Part model, mm, in its own coordinate system. A direction names the side the tool comes from. Give positions to 0.01 mm unless a question says otherwise; leave off trailing zeros. Order: outer loops, then holes, each group sorted by start corner. A loop starts at its lowest first (then second) coordinate and runs counter-clockwise, first axis right, second up. Notation, with made-up numbers: M 33.25,29.5 L 83.25,29.5 A17 ccw 83.25,35.5 Z; hole C -4,34 d6. An arc over 180 degrees is marked long. Answer as a JSON object with one key per item and string values.
from build123d import *

# Parameters (mm, degrees)
BOSS_EXTRUDE1_DEPTH = 2.54
SKETCH2_R           = 6.35
CUT_EXTRUDE1_DEPTH  = 2.54
SKETCH3_W           = 175.067056309
SKETCH3_H           = 2.54
BOSS_EXTRUDE2_DEPTH = 7.62
SKETCH4_W           = 175.067056309
SKETCH4_H           = 29.21
SKETCH4_W_2         = 164.016975536
SKETCH4_H_2         = 66.475239383
SKETCH4_W_3         = 84.822418372
SKETCH4_H_3         = 89.286756182
CUT_EXTRUDE2_DEPTH  = 2.54
FILLET1_R           = 12.7


with BuildPart() as part:
    # Sketch1 → Boss-Extrude1 (new body)
    with BuildSketch(Plane.XY.offset(-12.457776114)):
        Polygon((-175.067056309, 77.80274772), (129.732943691, 77.80274772), (129.732943691, 21.857628122), (0, 21.857628122), (0, -19.695936064), (-175.067056309, -19.695936064), align=None)
        with BuildLine():
            Line((-152.479240823, 20.309063936), (-5.464407031, 20.309063936))
            ThreePointArc((-5.464407031, 20.309063936), (-3.559407031, 18.404063936), (-5.464407031, 16.499063936))
            Line((-5.464407031, 16.499063936), (-152.479240823, 16.499063936))
            ThreePointArc((-152.479240823, 16.499063936), (-154.384240823, 18.404063936), (-152.479240823, 20.309063936))
        make_face(mode=Mode.SUBTRACT)
    extrude(amount=-BOSS_EXTRUDE1_DEPTH)

    # Sketch2 → Cut-Extrude1 (cut)
    with BuildSketch(Plane.XY.offset(-12.457776114)):
        with Locations((22.439796045, 50.825535486)):
            Circle(SKETCH2_R)
    extrude(amount=-CUT_EXTRUDE1_DEPTH, mode=Mode.SUBTRACT)

    # Sketch3 → Boss-Extrude2 (add)
    with BuildSketch(Plane.XY.offset(-12.457776114)):
        with Locations((-87.533528155, 26.024063936)):
            Rectangle(SKETCH3_W, SKETCH3_H)
        with Locations((-87.533528155, 10.784063936)):
            Rectangle(SKETCH3_W, SKETCH3_H)
    extrude(amount=BOSS_EXTRUDE2_DEPTH)

    # Sketch4 → Cut-Extrude2 (cut)
    with BuildSketch(Plane.XY.offset(-12.457776114)):
        with Locations((-87.533528155, -5.090936064)):
            Rectangle(SKETCH4_W, SKETCH4_H)
        with Locations((-93.058568541, 60.531683628)):
            Rectangle(SKETCH4_W_2, SKETCH4_H_2)
        with Locations((90.924098408, 47.502895008)):
            Rectangle(SKETCH4_W_3, SKETCH4_H_3)
    extrude(amount=-CUT_EXTRUDE2_DEPTH, mode=Mode.SUBTRACT)

    # Fillet1
    # the kernel refuses this fillet: 12.7 mm, written as the material it adds along each edge
    with BuildSketch(Plane(origin=(-11.050080773, 27.294063936, -12.457776114), x_dir=(0, 1, 0), z_dir=(0, 0, -1))) as fillet1_piece_1:
        with BuildLine():
            CenterArc((FILLET1_R, -FILLET1_R), FILLET1_R, 90, 90)
            Line((0, -FILLET1_R), (0, 0))
            Line((0, 0), (FILLET1_R, 0))
        make_face()
    extrude(amount=2.54)
    with BuildSketch(Plane(origin=(0, 21.857628122, 19.279716847), x_dir=(0, -1, 0), z_dir=(0, 0, -1))) as fillet1_piece_2_section:
        with BuildLine():
            CenterArc((12.7, -12.694997184), FILLET1_R, 91.608263763, 88.391736237)
            Line((0, -12.694997184), (0, 0))
            Line((0, 0), (12.343564187, 0))
        make_face()
    fillet1_piece_2 = extrude(amount=34.277492961, mode=Mode.PRIVATE)
    fillet1_piece_2 = split(fillet1_piece_2, bisect_by=Plane(origin=(0, 12.054063936, 19.279716847), z_dir=(0, -1, 0)), keep=Keep.TOP, mode=Mode.PRIVATE)
    fillet1_piece_2 = split(fillet1_piece_2, bisect_by=Plane(origin=(0, 21.857628122, -4.837776114), z_dir=(0, 0, -1)), keep=Keep.TOP, mode=Mode.PRIVATE)
    add(fillet1_piece_2)
    with BuildSketch(Plane(origin=(0, 21.857628122, -12.457776114), x_dir=(0, -1, 0), z_dir=(0, 0, -1))) as fillet1_piece_3:
        with BuildLine():
            CenterArc((12.7, -12.694997184), FILLET1_R, 91.608263763, 88.391736237)
            Line((0, -12.694997184), (0, 0))
            Line((0, 0), (12.343564187, 0))
        make_face()
    extrude(amount=2.54)
    # the kernel refuses this fillet: 12.7 mm, written as the material it takes off along each edge
    with BuildSketch(Plane(origin=(48.512889222, 21.857628122, -46.747776114), x_dir=(-1, 0, 0), z_dir=(0, 0, 1)), Plane(origin=(48.512889222, 77.80274772, 19.292223886), x_dir=(-1, 0, 0), z_dir=(0, 0, -1)), Plane(origin=(-11.050080773, 77.80274772, -46.747776114), x_dir=(1, 0, 0), z_dir=(0, 0, 1))) as fillet1_2_piece_1:
        with BuildLine():
            CenterArc((FILLET1_R, -FILLET1_R), FILLET1_R, 90, 90)
            Line((0, -FILLET1_R), (0, 0))
            Line((0, 0), (FILLET1_R, 0))
        make_face()
    extrude(amount=66.04, mode=Mode.SUBTRACT)


solid = part.part
1. Two-plate mould, pull along X, no slides. Class faces 1 (the flat face through (-39, 26, -14.998)), 2 (the cylindrical face through (17.76, 55.12, -13.71)), 3 (the cylindrical face through (-7.23, 74.18, -13.75)): +X half, -X half, draft (parallel to the pull), parting line (faces both ways), or undercut.
Worked answers:
{"face 1": "draft", "face 2": "undercut", "face 3": "-X half"}
2. Cut at A-A on z = -8. Give the cut face in (x, y) (3 decimals), plus the area to 3 significant figures.
Worked answers:
{"outline": "M -175.067,9.514 L 0,9.514 A12.7 cw 0.33,12.054 L -175.067,12.054 Z; M -175.067,24.754 L 0,24.754 L 0,27.294 L -175.067,27.294 Z", "area": "890 mm^2"}
3. Which spindle directions (+Z, -Z, +X, -X, +Y, -Y) get a long thin tool onto all of the face, cutting with end or side? Do faces 4 (the cylindrical face through (-14.672, 31.113, -13.71)), 5 (the flat face through (-89, 24.754, -9)). Say none if no direction does.
Worked answers:
{"face 4": "+Z, -Z, -X, +Y", "face 5": "+Z, +X, -X"}
4. Cut at D-D on x = -14. Give the cut face in (y, z), plus the area to 3 significant figures.
Worked answers:
{"outline": "M 9.51,-15 L 16.5,-15 L 16.5,-12.46 L 12.05,-12.46 L 12.05,-4.84 L 9.51,-4.84 Z; M 20.31,-15 L 31.86,-15 L 31.86,-12.46 L 27.29,-12.46 L 27.29,-4.84 L 24.75,-4.84 L 24.75,-12.46 L 20.31,-12.46 Z", "area": "85.8 mm^2"}
5. Cut at C-C on y = 47. Give the cut face in (x, z).
Worked answers:
{"outline": "M -11.05,-15 L 17.37,-15 L 17.37,-12.46 L -11.05,-12.46 Z; M 27.51,-15 L 48.51,-15 L 48.51,-12.46 L 27.51,-12.46 Z"}
6. Cut at B-B on x = -44. Give the cut face in (y, z), plus the area to 3 significant figures.
Worked answers:
{"outline": "M 9.51,-15 L 16.5,-15 L 16.5,-12.46 L 12.05,-12.46 L 12.05,-4.84 L 9.51,-4.84 Z; M 20.31,-15 L 27.29,-15 L 27.29,-4.84 L 24.75,-4.84 L 24.75,-12.46 L 20.31,-12.46 Z", "area": "74.2 mm^2"}
7. Probe line 1 along Y through (x, z) = (-69, -9.25); line 2 along Y through (x, z) = (-40, -14); line 3 along Z through (x, y) = (36, 54). List the from-to ranges inside material, lowest first.
Worked answers:
{"line 1": "y = 9.51 to 12.05, 24.75 to 27.29", "line 2": "y = 9.51 to 16.5, 20.31 to 27.29", "line 3": "z = -15 to -12.46"}
8. Pin check, flat tips, straight feed: P1, Ø3, axis at x = -128.5, z = -8, coming from the +Y side; P2, Ø0.8, axis at y = 52.5, z = -14, coming from the -X side; P3, Ø6, axis at x = -6.5, y = 32, coming from the +Z side. Stop position of each tip, or through.
Worked answers:
{"P1": "stops at y = 27.29", "P2": "stops at x = -11.05", "P3": "stops at z = -12.46"}
